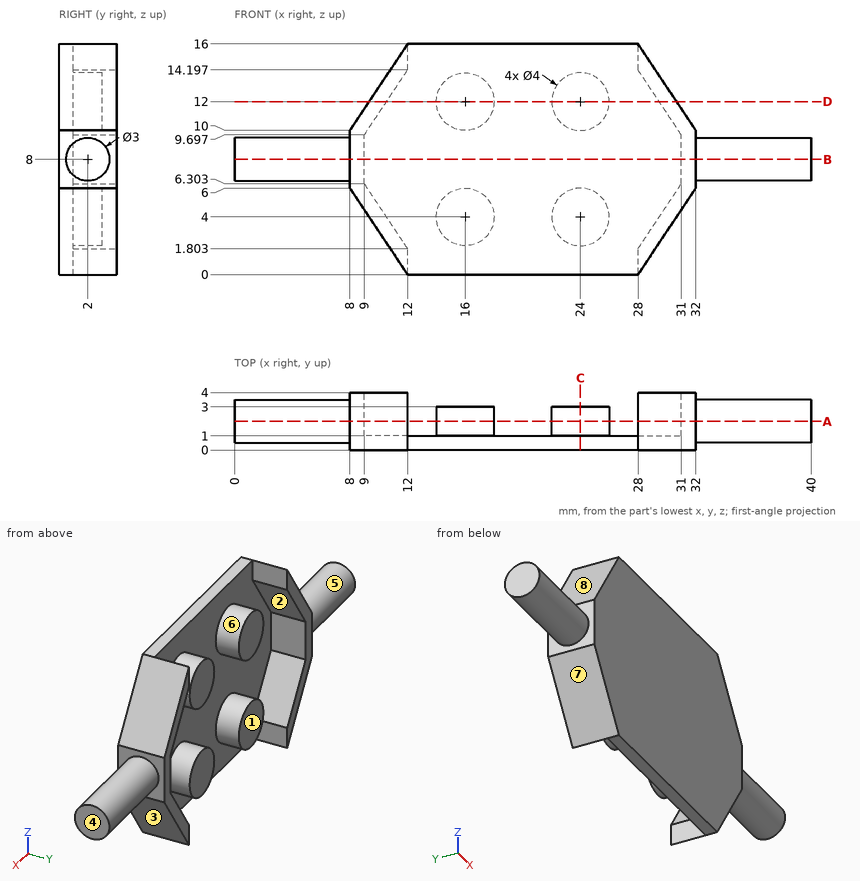
Geometry: see drawing. Coordinates: mm, zero at the bounding-box minimum. A direction names the side the tool comes from. Coordinates: 2 decimals unless noted, no trailing zeros. Write each loop counter-clockwise with the first axis right and the second up, starting at its lowest first coordinate (ties: lowest second). Pieces come first, ordered by that corner, then holes.
1) Section C-C on x = 24. Output: boundary loops of the cut face in (y, z).
2) Section B-B on z = 8. Output: boundary loops of the cut face in (x, y), and give its area (3 significant figures).
3) Set-up query: the marked faces 1, 2, 3, 4 and 5. Return all of +Z, -Z, +X, -X, +Y, -Y with unobstructed straight access to the full face (end or side cutting, diameter ignored); none if empty.
4) Material intervals for line 1 along X through (y, z) = (1.45, 11.5); line 2 along X through (y, z) = (2, 8.5); line 3 along X through (y, z) = (2.6, 11.75) (1 decimal), sorted ascending.
5) Pin query (flat end, axial travel): pin 1 Ø2 at (y, z) = (2, 1.5) entering from +X; pin 2 Ø0.5 at (y, z) = (2, 15.5) entering from +X; pin 3 Ø0.5 at (y, z) = (2, 15.5) entering from -X. Return the tip coordinate at first contact, or that it passes through.
6) Section D-D on z = 12. Output: boundary loops of the cut face in (x, y) (1 decimal).
7) Section A-A on y = 2. Output: boundary loops of the cut face in (x, z), and give its area (3 significant figures).
8) Mould query, pull axis Z, two halves, no side actions, for the marked faces 6, 7 and 8. Classes: pulls with the +Z half, pulls with the -Z half, needs draft (parallel to the pull), parting line crosses it, or undercut.
Check result:
1. outline: (0, 0) - (1, 0) - (1, 2) - (3, 2) - (3, 6) - (1, 6) - (1, 10) - (3, 10) - (3, 14) - (1, 14) - (1, 16) - (0, 16) - close
2. outline: (0, 0.5) - (8, 0.5) - (8, 0) - (32, 0) - (32, 0.5) - (40, 0.5) - (40, 3.5) - (32, 3.5) - (32, 4) - (31, 4) - (31, 1) - (9, 1) - (9, 4) - (8, 4) - (8, 3.5) - (0, 3.5) - close
2. area: 78.0 mm2
3. face 1: +Z, -Z, +Y
3. face 2: +Y
3. face 3: -Z, +X, +Y, -Y
3. face 4: +Z, -Z, +X, +Y, -Y
3. face 5: -X
4. line 1: x = 9 to 10.2, 14.06 to 17.94, 22.06 to 25.94, 29.8 to 31
4. line 2: x = 0 to 9, 31 to 40
4. line 3: x = 9.2 to 10.4, 14 to 18, 22 to 26, 29.6 to 30.8
5. pin 1: stops at x = 29.67
5. pin 2: stops at x = 28.5
5. pin 3: stops at x = 11.5
6. outline: (9.3, 0) - (30.7, 0) - (30.7, 4) - (29.5, 4) - (29.5, 1) - (26, 1) - (26, 3) - (22, 3) - (22, 1) - (18, 1) - (18, 3) - (14, 3) - (14, 1) - (10.5, 1) - (10.5, 4) - (9.3, 4) - close
7. outline: (0, 6.5) - (8, 6.5) - (8, 6) - (12, 0) - (12, 1.8) - (9, 6.3) - (9, 9.7) - (12, 14.2) - (12, 16) - (8, 10) - (8, 9.5) - (0, 9.5) - close; circle Ø4 at (16, 4); circle Ø4 at (16, 12); circle Ø4 at (24, 4); circle Ø4 at (24, 12); (28, 0) - (32, 6) - (32, 6.5) - (40, 6.5) - (40, 9.5) - (32, 9.5) - (32, 10) - (28, 16) - (28, 14.2) - (31, 9.7) - (31, 6.3) - (28, 1.8) - close
7. area: 131 mm2
8. face 6: undercut
8. face 7: pulls with the -Z half
8. face 8: pulls with the +Z half
